from build123d import *

# Parameters (mm, degrees)
SKETCH_W     = 24.5
SKETCH_H     = 11.1
SKETCH_W_2   = 20.5
SKETCH_H_2   = 7.1
PAD_DEPTH    = 6.7
SKETCH001_W  = 90
SKETCH001_H  = 17.3
PAD001_DEPTH = 0.5


with BuildPart() as part:
    # Sketch (on Sketch) → Pad (new body)
    with BuildSketch(Plane.XY):
        Rectangle(SKETCH_W, SKETCH_H)
        Rectangle(SKETCH_W_2, SKETCH_H_2, mode=Mode.SUBTRACT)
    extrude(amount=PAD_DEPTH)

    # Sketch001 → Pad001 (join)
    with BuildSketch(Plane.XY):
        with Locations((-32.851308, 0)):
            Rectangle(SKETCH001_W, SKETCH001_H)
    extrude(amount=-PAD001_DEPTH)


solid = part.part
Work out the finished part from the listing and answer in its coordinate system (mm). A direction names the side the tool comes from. Coordinates: 2 decimals unless noted, no trailing zeros. Loops run counter-clockwise (first coordinate to the right, second up) from the corner with the lowest first, then second, coordinate; pieces in that order, holes last. Notation, with made-up numbers: (-24.5, 65) -> (-16.5, 65) arc R32 cw to (-16.5, 97) -> close; hole circle Ø3 at (-6.75, 79.5). An arc over 180 degrees is marked (long way). Answer as CSV lines item,"result".
1) The part is cut by section B-B (x = 6). Give the vertices of the cut face in (y, z), and give its area (4 significant figures).
A:
outline,"(-8.65, -0.5) -> (8.65, -0.5) -> (8.65, 0) -> (5.55, 0) -> (5.55, 6.7) -> (3.55, 6.7) -> (3.55, 0) -> (-3.55, 0) -> (-3.55, 6.7) -> (-5.55, 6.7) -> (-5.55, 0) -> (-8.65, 0) -> close"
area,"35.45 mm²"
2) For faces 4 (the face through (-12.25, 0, 3)), 5 (the face through (-33, 0, -0.5)), 6 (the face through (0, -5.55, 3)), 7 (the face through (-10.25, 0, 3)), determine the directions among +Z, -Z, +X, -X, +Y, -Y from which every point of the face is accessible in a straight line to the end or side of a thin tool.
A:
face 4,"+Z, -X, +Y, -Y"
face 5,"-Z, +X, -X, +Y, -Y"
face 6,"+Z, +X, -X, -Y"
face 7,"+Z"
3) The part is cut by section C-C (y = 1). Give the vertices of the cut face in (x, z), and give its area (3 significant figures).
A:
outline,"(-77.85, -0.5) -> (12.15, -0.5) -> (12.15, 0) -> (12.25, 0) -> (12.25, 6.7) -> (10.25, 6.7) -> (10.25, 0) -> (-10.25, 0) -> (-10.25, 6.7) -> (-12.25, 6.7) -> (-12.25, 0) -> (-77.85, 0) -> close"
area,"71.8 mm²"
4) Straight lines are drawn through the part: probe 1 along X at (y, z) = (-0.25, 1); probe 2 along Y at (x, z) = (-9, 5); probe 3 along X at (y, z) = (-5.5, 2). For each, find the intervals that lie inside material, in ascending order.
A:
probe 1,"x = -12.25 to -10.25, 10.25 to 12.25"
probe 2,"y = -5.55 to -3.55, 3.55 to 5.55"
probe 3,"x = -12.25 to 12.25"
5) Flat-ended cylindrical pins translate along their axes: pin 1 (3.5 mm diameter, centred on y = 1, z = 4, fed in from -X); pin 2 (2 mm diameter, centred on x = 2, z = 4.5, fed in from -Y); pin 3 (3.5 mm diameter, centred on x = 4.5, z = 3, fed in from +Y). Find the tip coordinate at first contact, or state that the pin passes through.
A:
pin 1,"stops at x = -12.25"
pin 2,"stops at y = -5.55"
pin 3,"stops at y = 5.55"
6) For a pull along Y with two mould halves and no side action, classify faces 1 (the face through (0, 5.55, 3)), 2 (the face through (0, 3.55, 3)), 3 (the face through (12.25, 0, 3)) as released by +Y, released by -Y, zero draft, split by the parting line, or undercut.
A:
face 1,"released by +Y"
face 2,"undercut"
face 3,"zero draft"
7) The part is cut by section A-A (z = 1.5). Give the vertices of the cut face in (x, y).
A:
outline,"(-12.25, -5.55) -> (12.25, -5.55) -> (12.25, 5.55) -> (-12.25, 5.55) -> close; hole (-10.25, -3.55) -> (10.25, -3.55) -> (10.25, 3.55) -> (-10.25, 3.55) -> close"
8) The part is cut by section D-D (x = -32). Give the vertices of the cut face in (y, z), and give its area (3 significant figures).
A:
outline,"(-8.65, -0.5) -> (8.65, -0.5) -> (8.65, 0) -> (-8.65, 0) -> close"
area,"8.65 mm²"
